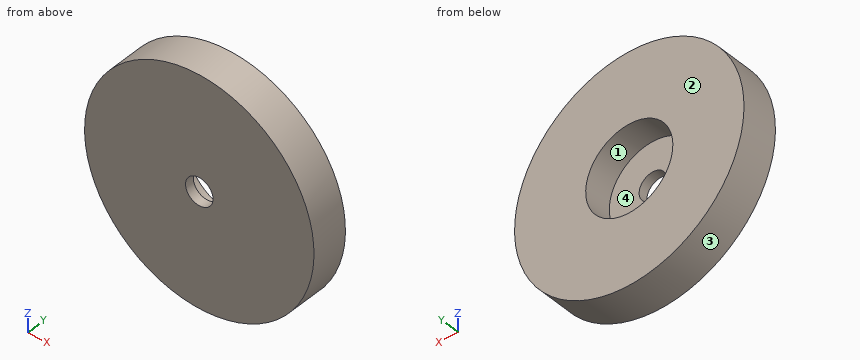
from build123d import *

# Parameters (mm, degrees)
ESQUISSE1_R                  = 25
BOSS_EXTRU_1_DEPTH           = 8
ESQUISSE2_R                  = 9.5
ENL_V_MAT_EXTRU_1_DEPTH      = 6
ENL_V_MAT_EXTRU_2_DEPTH      = 37.249137921
ENL_V_MAT_EXTRU_2_DEPTH_BACK = 37.249137921
ESQUISSE4_R                  = 3


with BuildPart() as part:
    # Esquisse1 → Boss.-Extru.1 (new body)
    with BuildSketch(Plane(origin=(0, 0, 0), x_dir=(1, 0, 0), z_dir=(0, 1, 0))):
        with Locations(Location((0, 0, 0), (0, 0, 270))):
            Circle(ESQUISSE1_R)
    extrude(amount=BOSS_EXTRU_1_DEPTH)

    # Esquisse2 → Enlèv. mat.-Extru.1 (cut)
    with BuildSketch(Plane(origin=(0, 8, 0), x_dir=(1, 0, 0), z_dir=(0, 1, 0))):
        with Locations(Location((0, 0, 0), (0, 0, 270))):
            Circle(ESQUISSE2_R)
    extrude(amount=-ENL_V_MAT_EXTRU_1_DEPTH, mode=Mode.SUBTRACT)

    # Esquisse4 → Enlèv. mat.-Extru.2 (cut, two sides: drawn at the far end of the back side and taken through both)
    with BuildSketch(Plane.XZ.offset(-ENL_V_MAT_EXTRU_2_DEPTH_BACK)):
        with Locations(Location((0, 0, 0), (0, 0, 90))):
            Circle(ESQUISSE4_R)
    extrude(amount=ENL_V_MAT_EXTRU_2_DEPTH + ENL_V_MAT_EXTRU_2_DEPTH_BACK, mode=Mode.SUBTRACT)


solid = part.part
The model under review builds one solid part; all positions refer to its coordinate system, in mm. Face numbers are marked on the shaded views. Give positions to 0.01 mm unless a question says otherwise; leave off trailing zeros. Order: outer loops, then holes, each group sorted by start corner. A loop starts at its lowest first (then second) coordinate and runs counter-clockwise, first axis right, second up. Notation, with made-up numbers: M -10.5,71 L 26.5,71 A33 ccw 26.5,99 Z; hole C 26.25,78.25 d6. An arc over 180 degrees is marked long. One line per question, with ' | ' between items. Start each with the question number.
1) Wall thickness on L1, parallel to X at y = 0.7, z = 0; L2, parallel to X at y = 4.5, z = -0.5 (3 decimals); L3, parallel to Y at x = -4, z = 7: over which ranges is each line inside the solid? List them lowest first. Write a range as from..to.
2) Consider section B-B, the plane z = 0. Give the boundary of the cut face in (x, y), then the cut area to 3 significant figures.
3) Consider section A-A, the plane x = 0. Give the boundary of the cut face in (y, z), then the cut area to 3 significant figures.
4) Mouldability with a two-part tool opening along X and no side actions: class the marked faces 1, 2, 3 and 4 as pulls with the +X half, pulls with the -X half, needs draft (parallel to the pull), parting line crosses it, or undercut.
5) Consider section D-D, the plane y = 6. Give the boundary of the cut face in (x, z).
6) Consider section C-C, the plane z = 8. Give the boundary of the cut face in (x, y), then the cut area to 3 significant figures.
7) Clearance check with flat-ended pins moving along their axes: P1, Ø1, axis at y = 3, z = -2, coming from the +X side; P2, Ø7, axis at x = 0, z = 0, coming from the +Y side; P3, Ø4, axis at y = 3.5, z = -3, coming from the -X side. State where each tip first meets the part, or that it passes through.
Found:
1) L1: x = -25..-3, 3..25 | L2: x = -24.995..-9.487, 9.487..24.995 | L3: y = 0..2
2) outline: M -25,0 L -3,0 L -3,2 L -9.5,2 L -9.5,8 L -25,8 Z; M 3,0 L 25,0 L 25,8 L 9.5,8 L 9.5,2 L 3,2 Z | area: 274 mm²
3) outline: M 0,-25 L 8,-25 L 8,-9.5 L 2,-9.5 L 2,-3 L 0,-3 Z; M 0,3 L 2,3 L 2,9.5 L 8,9.5 L 8,25 L 0,25 Z | area: 274 mm²
4) face 1: undercut | face 2: needs draft | face 3: parting line crosses it | face 4: undercut
5) outline: C 0,0 d50; hole C 0,0 d19
6) outline: M -23.69,0 L 23.69,0 L 23.69,8 L 5.12,8 L 5.12,2 L -5.12,2 L -5.12,8 L -23.69,8 Z | area: 317 mm²
7) P1: stops at x = 24.95 | P2: stops at y = 2 | P3: stops at x = -24.98
